Source: three-view drawing plus pictorial views. Frame: mm from the lowest corner of the part. A direction names the side the tool comes from. Give positions to 0.01 mm unless a question says otherwise; leave off trailing zeros. Loops run counter-clockwise (first coordinate to the right, second up) from the corner with the lowest first, then second, coordinate; pieces in that order, holes last. Notation, with made-up numbers: (46, 27) - (66, 27) arc R16 ccw to (66, 56) - close; hole circle Ø5 at (26.5, 14). An arc over 180 degrees is marked (long way). Answer as a JSON object with one key per item and string values. Group by question number.
(1) Access query for the marked faces 4 and 5. Directions: +Z, -Z, +X, -X, +Y, -Y. A direction counts if a zero-diameter tool reaches every point of the face in a straight line with its end or side. Return the directions, or none.
(2) Pin query (flat end, axial travel): P1, Ø1.5, axis at y = 21.5, z = 14.5, coming from the -X side; P2, Ø4, axis at x = 32.5, y = 16.5, coming from the +Z side; P3, Ø2, axis at x = 59.5, z = 25, coming from the -Y side. Return the tip coordinate at first contact, or that it passes through.
(3) Material intervals for L1, parallel to Z at x = 35, y = 19.25; L2, parallel to X at y = 21.75, z = 18.5; L3, parallel to X at y = 23.75, z = 15.75, sorted ascending.
(4) Section query D-D (x = 15). Return loops of the section in (y, z).
(5) Section query C-C (z = 9.5). Return loops of the section in (x, y).
(6) Section query A-A (y = 15). Return loops of the section in (x, z), plus the area to 4 significant figures.
(7) Mould query, pull axis X, two halves, no side actions, for the marked faces 1, 2 and 3. Classes: +X half, -X half, draft (parallel to the pull), parting line (faces both ways), or undercut.
(8) Section query B-B (x = 54). Return loops of the section in (y, z), plus the area to 3 significant figures.
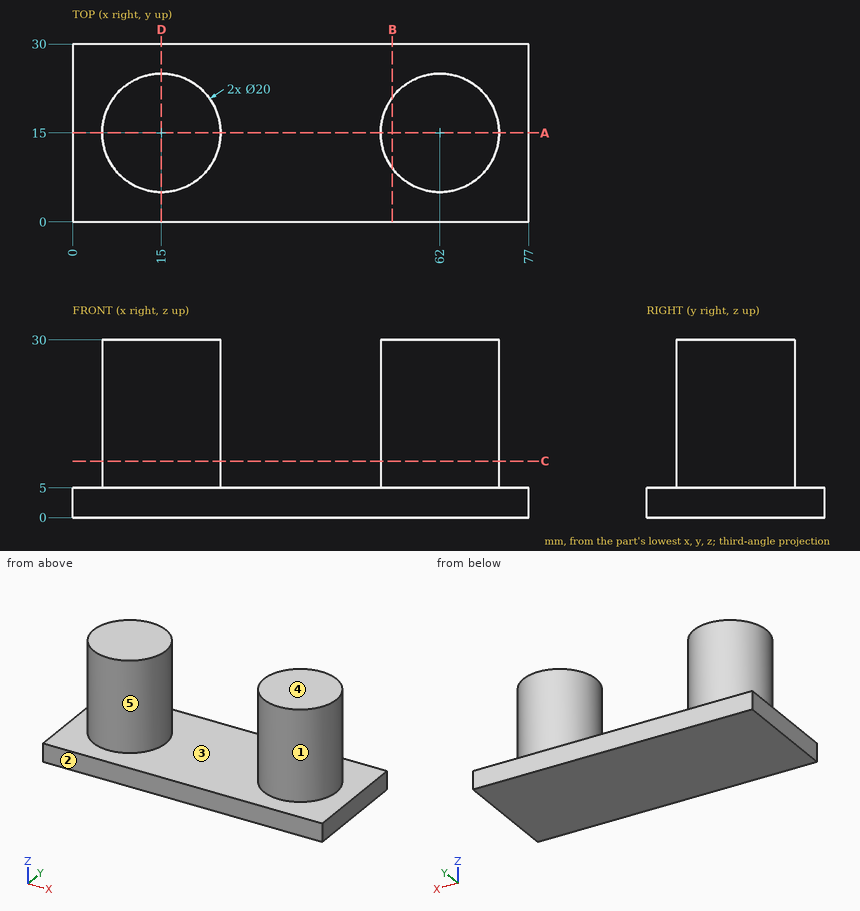
Recorded:
{
 "1": {"face 4": "+Z, +X, -X, +Y, -Y", "face 5": "+Z"},
 "2": {"P1": "stops at x = 6.82", "P2": "stops at z = 5", "P3": "stops at y = 5.11"},
 "3": {"L1": "z = 0 to 5", "L2": "x = 7.62 to 22.38, 54.62 to 69.38", "L3": "x = 10.16 to 19.84, 57.16 to 66.84"},
 "4": {"outline": "(0, 0) - (30, 0) - (30, 5) - (25, 5) - (25, 30) - (5, 30) - (5, 5) - (0, 5) - close"},
 "5": {"outline": "circle Ø20 at (15, 15); circle Ø20 at (62, 15)"},
 "6": {"outline": "(0, 0) - (77, 0) - (77, 5) - (72, 5) - (72, 30) - (52, 30) - (52, 5) - (25, 5) - (25, 30) - (5, 30) - (5, 5) - (0, 5) - close", "area": "1,385 mm^2"},
 "7": {"face 1": "undercut", "face 2": "draft", "face 3": "undercut"},
 "8": {"outline": "(0, 0) - (30, 0) - (30, 5) - (21, 5) - (21, 30) - (9, 30) - (9, 5) - (0, 5) - close", "area": "450 mm^2"}
}
